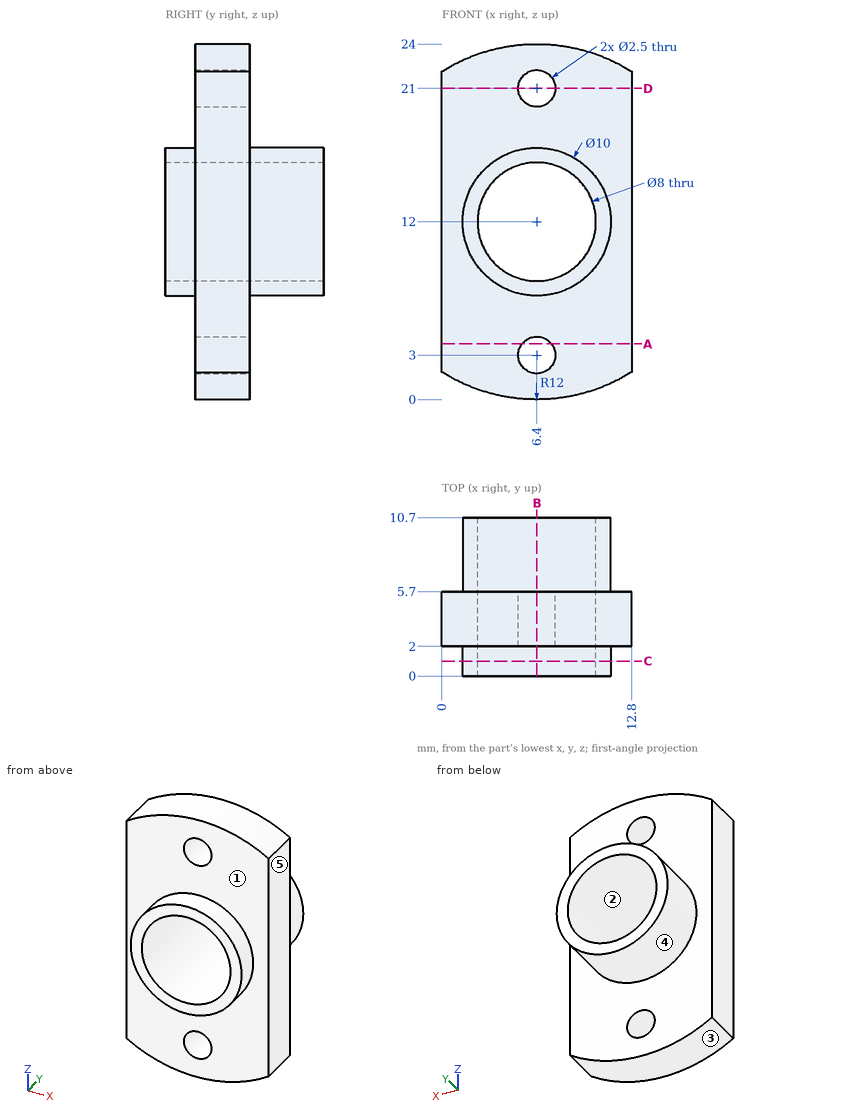
Drawing for the job (mm, zero at the part's lowest x, y, z). A direction names the side the tool comes from. Round coordinates to 2 decimals unless told otherwise and drop trailing zeros. Loops run counter-clockwise (first coordinate to the right, second up) from the corner with the lowest first, then second, coordinate; pieces in that order, holes last. Notation, with made-up numbers: (-20.5, -37) - (2.5, -37) arc R28 ccw to (2.5, -3) - close; hole circle Ø4 at (76.5, -16). An arc over 180 degrees is marked (long way). Return JSON: item names as keys, results as strings. Group by question number.
Q1. Two-plate mould, pull along Z, no slides. Class the marked faces 1, 2 and 3: +Z half, -Z half, draft (parallel to the pull), parting line (faces both ways), or undercut.
Q2. Flat gauge pins, fed straight in: pin 1 Ø3 at (x, z) = (6.4, 3) entering from +Y; pin 2 Ø2 at (x, z) = (6.4, 21) entering from +Y; pin 3 Ø5 at (x, y) = (11, 4) entering from +Z. Where does each tip first touch, or does it go through?
Q3. Drill centre lines: line 1 along Z through (x, y) = (6.5, 10); line 2 along Z through (x, y) = (6.75, 5.5); line 3 along X through (y, z) = (3.8, 3). Where is each one in solid material? Low to high. Write a range as [from, to].
Q4. Band-saw the part on A-A on z = 3.75. Give the cut face in (x, y).
Q5. Band-saw the part on D-D on z = 21. Give the cut face in (x, y), plus the area to 3 significant figures.
Q6. Band-saw the part on C-C on y = 1. Give the cut face in (x, z), plus the area to 3 significant figures.
Q7. Band-saw the part on B-B on x = 6.4. Give the cut face in (y, z).
Q8. Tool access for the marked faces 4 and 5: list every direction of +Z, -Z, +X, -X, +Y, -Y with a clear straight run to the whole face (end or side of a thin tool).
Solutions:
{
 "1": {"face 1": "draft", "face 2": "undercut", "face 3": "-Z half"},
 "2": {"pin 1": "stops at y = 5.7", "pin 2": "passes through", "pin 3": "stops at z = 23.81"},
 "3": {"line 1": "z = [7, 8], [16, 17]", "line 2": "z = [0.01, 1.8], [4.2, 8.02], [15.98, 19.8], [22.2, 23.99]", "line 3": "x = [0, 5.15], [7.65, 12.8]"},
 "4": {"outline": "(0, 2) - (5.4, 2) - (5.4, 5.7) - (0, 5.7) - close; (7.4, 2) - (12.8, 2) - (12.8, 5.7) - (7.4, 5.7) - close"},
 "5": {"outline": "(0, 2) - (5.15, 2) - (5.15, 5.7) - (0, 5.7) - close; (7.65, 2) - (12.8, 2) - (12.8, 5.7) - (7.65, 5.7) - close", "area": "38.1 mm^2"},
 "6": {"outline": "circle Ø10 at (6.4, 12); hole circle Ø8 at (6.4, 12)", "area": "28.3 mm^2"},
 "7": {"outline": "(0, 7) - (2, 7) - (2, 4.25) - (5.7, 4.25) - (5.7, 7) - (10.7, 7) - (10.7, 8) - (0, 8) - close; (0, 16) - (10.7, 16) - (10.7, 17) - (5.7, 17) - (5.7, 19.75) - (2, 19.75) - (2, 17) - (0, 17) - close; (2, 0) - (5.7, 0) - (5.7, 1.75) - (2, 1.75) - close; (2, 22.25) - (5.7, 22.25) - (5.7, 24) - (2, 24) - close"},
 "8": {"face 4": "+Y", "face 5": "+Z, -Z, +X, +Y, -Y"}
}
